Here's how the part is built. I have some questions about the finished solid (model axes, mm). A direction names the side the tool comes from. Give positions to 0.01 mm unless a question says otherwise; leave off trailing zeros. Write each loop counter-clockwise with the first axis right and the second up, starting at its lowest first coordinate (ties: lowest second). Pieces come first, ordered by that corner, then holes. Notation, with made-up numbers: (29, 87) -> (75, 87) arc R12 ccw to (75, 110) -> close; hole circle Ø5 at (6, 76). An arc over 180 degrees is marked (long way). Return JSON: item names as keys, results as strings.
from build123d import *

# Parameters (mm, degrees)
SKETCH1_R           = 7.5
SKETCH1_W           = 6.85
SKETCH1_H           = 6.85
BOSS_EXTRUDE1_DEPTH = 4
SKETCH2_R           = 11
SKETCH2_R_2         = 7.5
BOSS_EXTRUDE2_DEPTH = 1


with BuildPart() as part:
    # Sketch1 → Boss-Extrude1 (new body, symmetric)
    with BuildSketch(Plane.XY):
        Circle(SKETCH1_R)
        Rectangle(SKETCH1_W, SKETCH1_H, mode=Mode.SUBTRACT)
    extrude(amount=BOSS_EXTRUDE1_DEPTH, both=True)

    # Sketch2 → Boss-Extrude2 (add)
    with BuildSketch(Plane(origin=(0, 0, -4), x_dir=(-1, 0, 0), z_dir=(0, 0, -1))):
        Circle(SKETCH2_R)
        Circle(SKETCH2_R_2, mode=Mode.SUBTRACT)
    extrude(amount=-BOSS_EXTRUDE2_DEPTH)


solid = part.part
1. Suppose I cut it at A-A, the plane x = 0. List the corners of the cut face in (y, z) for me (3 decimals).
Taken from the geometry:
{"outline": "(-11, -4) -> (-3.425, -4) -> (-3.425, 4) -> (-7.5, 4) -> (-7.5, -3) -> (-11, -3) -> close; (3.425, -4) -> (11, -4) -> (11, -3) -> (7.5, -3) -> (7.5, 4) -> (3.425, 4) -> close"}
2. Suppose I cut it at B-B, the plane z = 0.75. List the corners of the cut face in (x, y) for me (3 decimals), and give its area (3 significant figures).
Taken from the geometry:
{"outline": "circle Ø15 at (0, 0); hole (-3.425, -3.425) -> (3.425, -3.425) -> (3.425, 3.425) -> (-3.425, 3.425) -> close", "area": "130 mm²"}
3. For pin 1 Ø3 at (x, z) = (6, 1) entering from +Y; pin 2 Ø2 at (y, z) = (-1, -0.5) entering from +X; pin 3 Ø3 at (x, z) = (3, -2) entering from +Y, each with a flat end and sliding along its axis, tell me the tip position at first contact or that it passes through.
Taken from the geometry:
{"pin 1": "stops at y = 6", "pin 2": "stops at x = 7.5", "pin 3": "stops at y = 10.84"}
4. If I drill on line 1 (X direction, y = -0.25, z = -1.75) (3 decimals); line 2 (Y direction, x = -2, z = 1.5) (3 decimals), over which ranges is the centre line in solid material (lowest first)? Write a range as [from, to].
Taken from the geometry:
{"line 1": "x = [-7.496, -3.425], [3.425, 7.496]", "line 2": "y = [-7.228, -3.425], [3.425, 7.228]"}
5. Which directions (+Z, -Z, +X, -X, +Y, -Y) give clear straight access to the entire face, cutting with the end or side of a thin tool? Please do faces 1 (the face through (0, 3.425, 0)), 2 (the face through (-7.2, 2.6, -3)).
Taken from the geometry:
{"face 1": "+Z, -Z", "face 2": "+Z"}
6. If we mould it in two halves opening along Y, with no side actions, what happens to faces 3 (the face through (-7.493, 0.33, 0.549)), 4 (the face through (0, -5, -4)), 5 (the face through (-3.425, 0, 0))? For each: released by +Y, released by -Y, zero draft, split by the parting line, or undercut.
Taken from the geometry:
{"face 3": "split by the parting line", "face 4": "zero draft", "face 5": "undercut"}
7. Suppose I cut it at D-D, the plane y = -4.5. List the corners of the cut face in (x, z) for me.
Taken from the geometry:
{"outline": "(-10.04, -4) -> (10.04, -4) -> (10.04, -3) -> (6, -3) -> (6, 4) -> (-6, 4) -> (-6, -3) -> (-10.04, -3) -> close"}
